from build123d import *

# Parameters (mm, degrees)
SKETCH1_W           = 12.319
SKETCH1_H           = 6
BOSS_EXTRUDE1_DEPTH = 15.24
SKETCH1_3_W         = 12.319
SKETCH1_3_H         = 6
SKETCH1_3_W_2       = 2.54
BOSS_EXTRUDE2_DEPTH = 2.54
SKETCH2_W           = 2.9845
SKETCH2_H           = 3.175
CUT_EXTRUDE1_DEPTH  = 19.545589779


with BuildPart() as part:
    # Sketch1 → Boss-Extrude1 (new body)
    with BuildSketch(Plane(origin=(0, 0, 0), x_dir=(1, 0, 0), z_dir=(0, 1, 0))):
        Rectangle(SKETCH1_W, SKETCH1_H)
    extrude(amount=BOSS_EXTRUDE1_DEPTH)

    # Sketch1_3 → Boss-Extrude2 (add)
    with BuildSketch(Plane(origin=(0, 0, 0), x_dir=(1, 0, 0), z_dir=(0, 1, 0))):
        Rectangle(SKETCH1_3_W, SKETCH1_3_H)
        with Locations((7.4295, 0)):
            Rectangle(SKETCH1_3_W_2, SKETCH1_3_H)
        with Locations((-7.4295, 0)):
            Rectangle(SKETCH1_3_W_2, SKETCH1_3_H)
    extrude(amount=-BOSS_EXTRUDE2_DEPTH)

    # Sketch2 → Cut-Extrude1 (cut, through all)
    with BuildSketch(Plane(origin=(0, 0, -3), x_dir=(-1, 0, 0), z_dir=(0, 0, -1))):
        with Locations((-4.66725, 10.7625)):
            Rectangle(SKETCH2_W, SKETCH2_H)
        with Locations((4.66725, 10.7625)):
            Rectangle(SKETCH2_W, SKETCH2_H)
    extrude(amount=-CUT_EXTRUDE1_DEPTH, mode=Mode.SUBTRACT)


solid = part.part
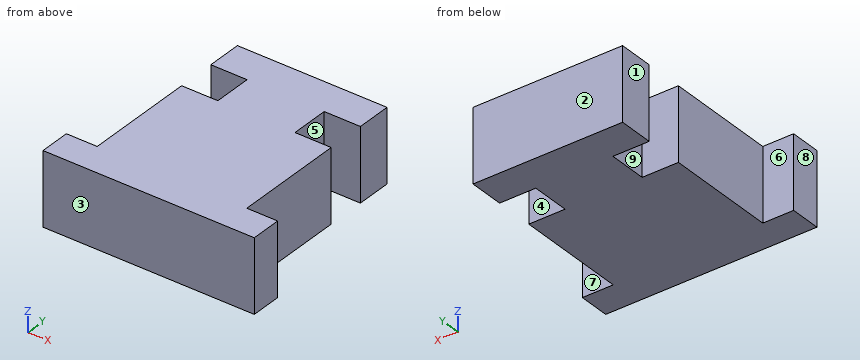
Work out the finished part from the listing and answer in its coordinate system (mm). Face numbers are marked on the shaded views. A direction names the side the tool comes from. Give positions to 0.01 mm unless a question says otherwise; leave off trailing zeros. Write each loop counter-clockwise with the first axis right and the second up, starting at its lowest first coordinate (ties: lowest second). Pieces come first, ordered by that corner, then holes. Notation, with made-up numbers: (78, -5.5) - (83, -5.5) arc R16 ccw to (83, 12.5) - close; hole circle Ø10 at (-32.75, 12). An arc over 180 degrees is marked (long way). One line per item, written item: value. Start each with the question number.
1. For a pull along Y with two mould halves and no side action, classify the marked faces 1, 2, 3 and 4 as +Y half, -Y half, draft (parallel to the pull), parting line (faces both ways), or undercut.
2. Find section A-A (x = 5.75). Write down the section's boundary in (y, z) (3 decimals).
3. For the marked faces 5, 6, 7, 8 and 9, determine the directions among +Z, -Z, +X, -X, +Y, -Y from which every point of the face is accessible in a straight line to the end or side of a thin tool.
4. Find section C-C (y = 5). Write down the section's boundary in (x, z), then the cut area to 3 significant figures.
5. Given pin 1 (0.8 mm diameter, centred on x = -7.5, z = 0, fed in from +Y); pin 2 (2.5 mm diameter, centred on y = 13.5, z = -0.5, fed in from +X); pin 3 (0.9 mm diameter, centred on y = 13.5, z = 0, fed in from -X), each flat-ended and moving along its own axis, determine where each tip first touches the part or whether it passes through.
6. Find section D-D (y = 11). Write down the section's boundary in (x, z) (3 decimals).
7. Consider probe 1 along Y at (x, z) = (-4.75, -0.85) (3 decimals); probe 2 along X at (y, z) = (4.75, -1.5); probe 3 along Y at (x, z) = (-6.75, 0.7). Determine where each line is inside the solid, lowest interval first.
Geometry results:
1. face 1: draft
1. face 2: +Y half
1. face 3: -Y half
1. face 4: undercut
2. outline: (-2.54, -3) - (9.175, -3) - (9.175, 3) - (-2.54, 3) - close; (12.35, -3) - (15.24, -3) - (15.24, 3) - (12.35, 3) - close
3. face 5: +Z, -Z, +X
3. face 6: +Z, -Z, -X, +Y
3. face 7: +Z, -Z, +X, +Y
3. face 8: +Z, -Z, -X, +Y, -Y
3. face 9: +Z, -Z, -X
4. outline: (-6.16, -3) - (6.16, -3) - (6.16, 3) - (-6.16, 3) - close
4. area: 73.9 mm2
5. pin 1: y = 0
5. pin 2: x = 6.16
5. pin 3: x = -6.16
6. outline: (-3.175, -3) - (3.175, -3) - (3.175, 3) - (-3.175, 3) - close
7. probe 1: -2.54 to 9.175, 12.35 to 15.24
7. probe 2: -6.16 to 6.16
7. probe 3: -2.54 to 0
